```python
from build123d import *

# Parameters (mm, degrees)
SKETCH1_R           = 57.5
SKETCH1_R_2         = 2
BOSS_EXTRUDE1_DEPTH = 5
SKETCH2_R           = 15
CUT_EXTRUDE1_DEPTH  = 1
SKETCH3_R           = 19
SKETCH3_R_2         = 15
BOSS_EXTRUDE3_DEPTH = 8


with BuildPart() as part:
    # Sketch1 → Boss-Extrude1 (new body)
    # profile 1 of 6: a face of its own
    with BuildSketch(Plane.XY):
        Circle(SKETCH1_R)
        with BuildLine():
            ThreePointArc((-52.440442409, 2.5), (-37.123106012, 37.123106012), (-2.5, 52.440442409))
            Line((-2.5, 52.440442409), (-2.5, 18.834808202))
            ThreePointArc((-2.5, 18.834808202), (0, 19), (2.5, 18.834808202))
            Line((2.5, 18.834808202), (2.5, 52.440442409))
            ThreePointArc((2.5, 52.440442409), (37.123106012, 37.123106012), (52.440442409, 2.5))
            Line((52.440442409, 2.5), (18.834808202, 2.5))
            ThreePointArc((18.834808202, 2.5), (18.958657071, 1.252725861), (19, 0))
            ThreePointArc((19, 0), (18.958657071, -1.252725861), (18.834808202, -2.5))
            Line((18.834808202, -2.5), (52.440442409, -2.5))
            ThreePointArc((52.440442409, -2.5), (37.123106012, -37.123106012), (2.5, -52.440442409))
            Line((2.5, -52.440442409), (2.5, -18.834808202))
            ThreePointArc((2.5, -18.834808202), (0, -19), (-2.5, -18.834808202))
            Line((-2.5, -18.834808202), (-2.5, -52.440442409))
            ThreePointArc((-2.5, -52.440442409), (-37.123106012, -37.123106012), (-52.440442409, -2.5))
            Line((-52.440442409, -2.5), (-18.834808202, -2.5))
            ThreePointArc((-18.834808202, -2.5), (-19, 0), (-18.834808202, 2.5))
            Line((-18.834808202, 2.5), (-52.440442409, 2.5))
        make_face(mode=Mode.SUBTRACT)
    # profile 2 of 6: a face of its own
    with BuildSketch(Plane.XY):
        with BuildLine():
            Line((-2.5, 14.790199458), (-2.5, 18.834808202))
            ThreePointArc((-2.5, 18.834808202), (-13.435028843, 13.435028843), (-18.834808202, 2.5))
            Line((-18.834808202, 2.5), (-14.790199458, 2.5))
            ThreePointArc((-14.790199458, 2.5), (-10.606601718, 10.606601718), (-2.5, 14.790199458))
        make_face()
    # profile 3 of 6: a face of its own
    with BuildSketch(Plane.XY):
        with BuildLine():
            Line((-14.790199458, -2.5), (-18.834808202, -2.5))
            ThreePointArc((-18.834808202, -2.5), (-13.435028843, -13.435028843), (-2.5, -18.834808202))
            Line((-2.5, -18.834808202), (-2.5, -14.790199458))
            ThreePointArc((-2.5, -14.790199458), (-10.606601718, -10.606601718), (-14.790199458, -2.5))
        make_face()
    # profile 4 of 6: a face of its own
    with BuildSketch(Plane.XY):
        with BuildLine():
            ThreePointArc((2.5, 18.834808202), (0, 19), (-2.5, 18.834808202))
            Line((-2.5, 18.834808202), (-2.5, 14.790199458))
            ThreePointArc((-2.5, 14.790199458), (-10.606601718, 10.606601718), (-14.790199458, 2.5))
            Line((-14.790199458, 2.5), (-18.834808202, 2.5))
            ThreePointArc((-18.834808202, 2.5), (-19, 0), (-18.834808202, -2.5))
            Line((-18.834808202, -2.5), (-14.790199458, -2.5))
            ThreePointArc((-14.790199458, -2.5), (-10.606601718, -10.606601718), (-2.5, -14.790199458))
            Line((-2.5, -14.790199458), (-2.5, -18.834808202))
            ThreePointArc((-2.5, -18.834808202), (0, -19), (2.5, -18.834808202))
            Line((2.5, -18.834808202), (2.5, -14.790199458))
            ThreePointArc((2.5, -14.790199458), (10.606601718, -10.606601718), (14.790199458, -2.5))
            Line((14.790199458, -2.5), (18.834808202, -2.5))
            ThreePointArc((18.834808202, -2.5), (18.958657071, -1.252725861), (19, 0))
            ThreePointArc((19, 0), (18.958657071, 1.252725861), (18.834808202, 2.5))
            Line((18.834808202, 2.5), (14.790199458, 2.5))
            ThreePointArc((14.790199458, 2.5), (10.606601718, 10.606601718), (2.5, 14.790199458))
            Line((2.5, 14.790199458), (2.5, 18.834808202))
        make_face()
        Circle(SKETCH1_R_2, mode=Mode.SUBTRACT)
    # profile 5 of 6: a face of its own
    with BuildSketch(Plane.XY):
        with BuildLine():
            ThreePointArc((18.834808202, 2.5), (13.435028843, 13.435028843), (2.5, 18.834808202))
            Line((2.5, 18.834808202), (2.5, 14.790199458))
            ThreePointArc((2.5, 14.790199458), (10.606601718, 10.606601718), (14.790199458, 2.5))
            Line((14.790199458, 2.5), (18.834808202, 2.5))
        make_face()
    # profile 6 of 6: a face of its own
    with BuildSketch(Plane.XY):
        with BuildLine():
            ThreePointArc((2.5, -18.834808202), (13.435028843, -13.435028843), (18.834808202, -2.5))
            Line((18.834808202, -2.5), (14.790199458, -2.5))
            ThreePointArc((14.790199458, -2.5), (10.606601718, -10.606601718), (2.5, -14.790199458))
            Line((2.5, -14.790199458), (2.5, -18.834808202))
        make_face()
    extrude(amount=BOSS_EXTRUDE1_DEPTH)

    # Sketch2 → Cut-Extrude1 (cut)
    with BuildSketch(Plane.XY.offset(5)):
        Circle(SKETCH2_R)
    extrude(amount=-CUT_EXTRUDE1_DEPTH, mode=Mode.SUBTRACT)

    # Sketch3 → Boss-Extrude3 (add)
    with BuildSketch(Plane.XY.offset(5)):
        with Locations(Location((0, 0, 0), (0, 0, 172.439156823))):
            Circle(SKETCH3_R)
        Circle(SKETCH3_R_2, mode=Mode.SUBTRACT)
    extrude(amount=BOSS_EXTRUDE3_DEPTH)


solid = part.part
```
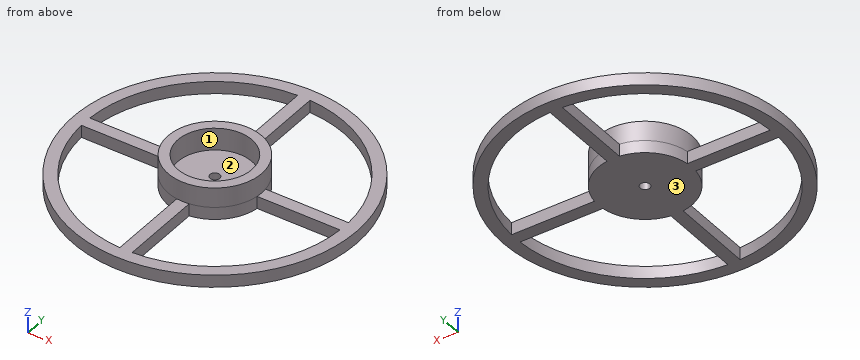
The listing builds one solid part. Answer for the finished solid, in the listing's coordinates (mm). Face numbers are marked on the shaded views. Round coordinates to 2 decimals unless told otherwise and drop trailing zeros. Order: outer loops, then holes, each group sorted by start corner. A loop starts at its lowest first (then second) coordinate and runs counter-clockwise, first axis right, second up. Notation, with made-up numbers: (-31, 62.25) -> (12, 62.25) arc R34 cw to (12, 98.25) -> close; hole circle Ø2 at (-16, -25.5). An arc over 180 degrees is marked (long way). Answer as CSV lines item,"result".
Q1. A cutting plane is placed at C-C on x = 26. Determine the outline of the cut face in (y, z), plus the area to 3 significant figures.
Computed values:
outline,"(-51.29, 0) -> (-45.61, 0) -> (-45.61, 5) -> (-51.29, 5) -> close; (-2.5, 0) -> (2.5, 0) -> (2.5, 5) -> (-2.5, 5) -> close; (45.61, 0) -> (51.29, 0) -> (51.29, 5) -> (45.61, 5) -> close"
area,"81.8 mm^2"
Q2. For a pull along X with two mould halves and no side action, classify the marked faces 1, 2 and 3 as +X half, -X half, draft (parallel to the pull), parting line (faces both ways), or undercut.
Computed values:
face 1,"undercut"
face 2,"undercut"
face 3,"draft"
Q3. A cutting plane is placed at D-D on z = 9.5. Determine the outline of the cut face in (x, y), plus the area to 3 significant figures.
Computed values:
outline,"circle Ø38 at (0, 0); hole circle Ø30 at (0, 0)"
area,"427 mm^2"
Q4. Consider line 1 (Y direction, x = 0, z = 2.9); line 2 (Y direction, x = -44, z = 1.5); line 3 (X direction, y = -12, z = 2.75). Determine where each line is inside the solid, lowest interval first. Write a range as from..to.
Computed values:
line 1,"y = -57.5..-2, 2..57.5"
line 2,"y = -37.02..-28.64, -2.5..2.5, 28.64..37.02"
line 3,"x = -56.23..-51.11, -14.73..14.73, 51.11..56.23"
Q5. A cutting plane is placed at A-A on y = 0. Determine the outline of the cut face in (x, z).
Computed values:
outline,"(-57.5, 0) -> (-2, 0) -> (-2, 4) -> (-15, 4) -> (-15, 13) -> (-19, 13) -> (-19, 5) -> (-57.5, 5) -> close; (2, 0) -> (57.5, 0) -> (57.5, 5) -> (19, 5) -> (19, 13) -> (15, 13) -> (15, 4) -> (2, 4) -> close"
Q6. Given pin 1 (6 mm diameter, centred on y = 29.5, z = 5, fed in from +X); pin 2 (2.5 mm diameter, centred on y = -39, z = 3, fed in from -X); pin 3 (4 mm diameter, centred on x = -31, z = 2.5, fed in from +Y), each flat-ended and moving along its own axis, determine where each tip first touches the part or whether it passes through.
Computed values:
pin 1,"stops at x = 51.03"
pin 2,"stops at x = -43.37"
pin 3,"stops at y = 49.65"
